from build123d import *

# Parameters (mm, degrees)
BOSS_EXTRUDE1_DEPTH = 25
FILLET1_R           = 2


with BuildPart() as part:
    # Sketch1 → Boss-Extrude1 (new body)
    with BuildSketch(Plane(origin=(0, 0, 0), x_dir=(-1, 0, 0), z_dir=(0, 1, 0))):
        with BuildLine():
            Line((1.837857672, 20.196095642), (2.372417379, 26.409673621))
            ThreePointArc((2.372417379, 26.409673621), (3.522331642, 28.481542299), (5.833566285, 29.004167449))
            ThreePointArc((5.833566285, 29.004167449), (11.321689347, 27.332975969), (16.384089207, 24.633997765))
            ThreePointArc((16.384089207, 24.633997765), (17.648827109, 22.630156287), (16.99690689, 20.352011723))
            Line((16.99690689, 20.352011723), (12.981234559, 15.580357805))
            ThreePointArc((12.981234559, 15.580357805), (11.222292108, 14.584351213), (9.239918516, 14.97944945))
            ThreePointArc((9.239918516, 14.97944945), (6.73522841, 16.260279772), (4.058461244, 17.125679325))
            ThreePointArc((4.058461244, 17.125679325), (2.377334792, 18.248052492), (1.837857672, 20.196095642))
        make_face()
    extrude(amount=BOSS_EXTRUDE1_DEPTH)

    # Fillet1
    fillet1_edges = [part.edges().sort_by_distance(p)[0] for p in [
        (-11.222292108, 25, 14.584351213),
        (-14.989070724, 25, 17.966184764),
        (-17.648827109, 25, 22.630156287),
        (-11.321689347, 25, 27.332975969),
        (-3.522331642, 25, 28.481542299),
        (-2.105137526, 25, 23.302884632),
        (-2.377334792, 25, 18.248052492),
        (-6.73522841, 25, 16.260279772),
    ]]
    fillet(fillet1_edges, radius=FILLET1_R)


solid = part.part
Geometry check sheet. Reference: the model listing, model coordinates, mm. Give positions to 0.01 mm unless a question says otherwise; leave off trailing zeros. Order: outer loops, then holes, each group sorted by start corner. A loop starts at its lowest first (then second) coordinate and runs counter-clockwise, first axis right, second up.
1. Sectioned sample at A-A (y = 6.25). Record the boundary of the cut face in (x, z) (3 decimals), then the cut area to 3 significant figures.
Completed:
outline: (-16.997, 20.352) - (-12.981, 15.58) arc R2.9 ccw to (-9.24, 14.979) arc R17.6 cw to (-4.058, 17.126) arc R2.9 ccw to (-1.838, 20.196) - (-2.372, 26.41) arc R2.9 ccw to (-5.834, 29.004) arc R29.585 ccw to (-16.384, 24.634) arc R2.9 ccw to start
area: 164 mm2
2. Scan lines: line 1 (Y direction, x = -13.5, z = 18.5); line 2 (Z direction, x = -13.75, y = 6.5); line 3 (Z direction, x = -8.75, y = 15.75). Record each from-to range of solid material in increasing order.
Completed:
line 1: y = 0 to 24.93
line 2: z = 16.49 to 26.2
line 3: z = 15.27 to 28.26
3. Depth check by flat-ended pin: pin 1 (2 mm diameter, centred on y = 16.5, z = 25, fed in from -X). Enter the tip coordinate at first touch or a pass-through.
Completed:
pin 1: stops at x = -17.07
